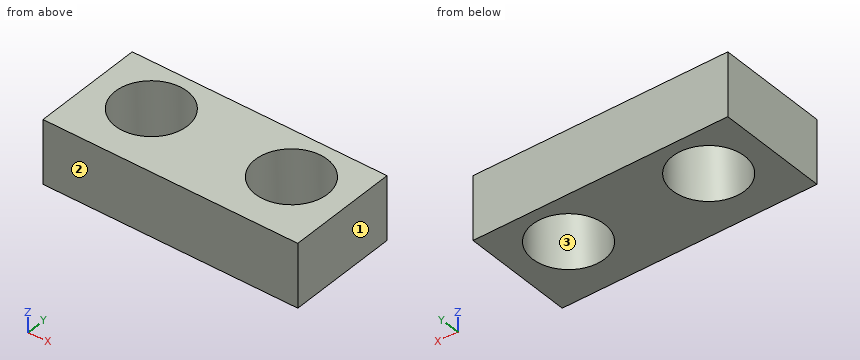
```python
from build123d import *

# Parameters (mm, degrees)
SKETCH1_W      = 8
SKETCH1_H      = 3.5
EXTRUDE1_DEPTH = 2
SKETCH2_R      = 1.1303
EXTRUDE2_DEPTH = 3


with BuildPart() as part:
    # Sketch1 → Extrude1 (new body)
    with BuildSketch(Plane.XY):
        with Locations((0, 1.25)):
            Rectangle(SKETCH1_W, SKETCH1_H)
    extrude(amount=-EXTRUDE1_DEPTH)

    # Sketch2 → Extrude2 (cut, through all)
    with BuildSketch(Plane.XY):
        with Locations((-2.2, 1.5)):
            Circle(SKETCH2_R)
        with Locations((2.2, 1.5)):
            Circle(SKETCH2_R)
    extrude(amount=-EXTRUDE2_DEPTH, mode=Mode.SUBTRACT)


solid = part.part
```
Read the model definition and answer for the solid it produces. Units are mm, in the model's axes. Face numbers are marked on the shaded views. Coordinates: 2 decimals unless noted, no trailing zeros. Loops run counter-clockwise (first coordinate to the right, second up) from the corner with the lowest first, then second, coordinate; pieces in that order, holes last. Notation, with made-up numbers: (-37.5, 29) - (16.5, 29) arc R21 cw to (16.5, 57) - close; hole circle Ø11 at (70.25, 86.5). An arc over 180 degrees is marked (long way). Answer in a Markdown table with one row per item.
1. Determine the mould class of the marked faces 1, 2 and 3 for opening direction X: +X half, -X half, draft (parallel to the pull), parting line (faces both ways), or undercut.
Conclusion:
| item | result |
|---|---|
| face 1 | +X half |
| face 2 | draft |
| face 3 | undercut |
2. Straight lines are drawn through the part: line 1 (Y direction, x = -2.2, z = -0.95); line 2 (X direction, y = 1.8, z = -1.5); line 3 (X direction, y = 0.7, z = -0.75). For each, find the intervals that lie inside material, in ascending order.
Conclusion:
| item | result |
|---|---|
| line 1 | y = -0.5 to 0.37, 2.63 to 3 |
| line 2 | x = -4 to -3.29, -1.11 to 1.11, 3.29 to 4 |
| line 3 | x = -4 to -3, -1.4 to 1.4, 3 to 4 |
3. Find section B-B, the plane y = 1.3. Write down the section's boundary in (x, z), then the cut area to 3 significant figures.
Conclusion:
| item | result |
|---|---|
| outline | (-4, -2) - (-3.31, -2) - (-3.31, 0) - (-4, 0) - close; (-1.09, -2) - (1.09, -2) - (1.09, 0) - (-1.09, 0) - close; (3.31, -2) - (4, -2) - (4, 0) - (3.31, 0) - close |
| area | 7.10 mm² |
4. Find section D-D, the plane y = 0.7. Write down the section's boundary in (x, z).
Conclusion:
| item | result |
|---|---|
| outline | (-4, -2) - (-3, -2) - (-3, 0) - (-4, 0) - close; (-1.4, -2) - (1.4, -2) - (1.4, 0) - (-1.4, 0) - close; (3, -2) - (4, -2) - (4, 0) - (3, 0) - close |
5. Find section A-A, the plane x = 2.2. Write down the section's boundary in (y, z).
Conclusion:
| item | result |
|---|---|
| outline | (-0.5, -2) - (0.37, -2) - (0.37, 0) - (-0.5, 0) - close; (2.63, -2) - (3, -2) - (3, 0) - (2.63, 0) - close |
6. Find section C-C, the plane z = -0.3. Write down the section's boundary in (x, y).
Conclusion:
| item | result |
|---|---|
| outline | (-4, -0.5) - (4, -0.5) - (4, 3) - (-4, 3) - close; hole circle Ø2.26 at (-2.2, 1.5); hole circle Ø2.26 at (2.2, 1.5) |
7. Given pin 1 (1.4 mm diameter, centred on x = 2.2, y = 1.5, fed in from -Z), flat-ended and moving along its own axis, determine where the tip first touches the part or whether it passes through.
Conclusion:
| item | result |
|---|---|
| pin 1 | passes through |
